from build123d import *

# Parameters (mm, degrees)
F2_R     = 3
F3_DEPTH = 50


with BuildPart() as f1:
    # F0 (on Front) → F1 (revolve)
    with BuildSketch(Plane.XZ):
        Polygon((0, 12.5), (0, 0), (22.5, 0), (22.5, 1), (10, 12.5), align=None)
        Polygon((0, 25), (0, 12.5), (10, 12.5), (16.372113, 25), align=None)
        Polygon((0, 37.5), (0, 25), (16.372113, 25), (10, 37.5), align=None)
        Polygon((0, 50), (0, 37.5), (10, 37.5), (22.5, 49), (22.5, 50), align=None)
    revolve(axis=Axis((0, 0, 25), (0, 0, 1)))

    # F2 (on face) → F3 (cut)
    with BuildSketch(Plane.XY.offset(50)):
        Circle(F2_R)
    extrude(amount=-F3_DEPTH, mode=Mode.SUBTRACT)


solid = f1.part
Design review of the part built by this model. Coordinates are the model's own, in mm. A direction names the side the tool comes from. Coordinates: 2 decimals unless noted, no trailing zeros. Loops run counter-clockwise (first coordinate to the right, second up) from the corner with the lowest first, then second, coordinate; pieces in that order, holes last. Notation, with made-up numbers: M 74,48.5 L 83,48.5 A27 cw 83,71.5 Z; hole C 61,-20.5 d5. An arc over 180 degrees is marked long. Answer as CSV lines item,"result".
Item 1: Add section D-D on z = 8.5. State the section outline as (x, y) points, plus the area to 3 significant figures.
Answer list:
outline,"C 0,0 d28.7; hole C 0,0 d6"
area,"618 mm²"
Item 2: Add section A-A on y = 0. State the section outline as (x, z) points, plus the area to 3 significant figures.
Answer list:
outline,"M -22.5,0 L -3,0 L -3,50 L -22.5,50 L -22.5,49 L -10,37.5 L -16.37,25 L -10,12.5 L -22.5,1 Z; M 3,0 L 22.5,0 L 22.5,1 L 10,12.5 L 16.37,25 L 10,37.5 L 22.5,49 L 22.5,50 L 3,50 Z"
area,"1,200 mm²"
Item 3: Add section C-C on y = 12. Count the separate pieces of the cut face and the enclosed holes in it, plus the area to 3 significant figures.
Answer list:
separate pieces,"3"
enclosed holes,"0"
area,"782 mm²"
Item 4: Machinability: for faces 1 (the face through (0, -5, 0)), 2 (the face through (-8.42, -6.45, 11.94)), which of the approach directions +Z, -Z, +X, -X, +Y, -Y give a long, thin tool a straight path to every point of the face, cutting with its end or side? Answer none if there is none.
Answer list:
face 1,"-Z, +X, -X, +Y, -Y"
face 2,"none"
Item 5: The part is to be moulded in two halves that separate along Z. For faces 3 (the face through (10.382, -19.961, 49.507)), 4 (the face through (-8.181, -6.273, 36.893)), 5 (the face through (-2.337, -10.526, 38.219)), 6 (the face through (0, -5, 50)), say which applies: pulls with the +Z half, pulls with the -Z half, needs draft (parallel to the pull), parting line crosses it, or undercut.
Answer list:
face 3,"needs draft"
face 4,"undercut"
face 5,"undercut"
face 6,"pulls with the +Z half"
Item 6: For P1, Ø1, axis at x = 5, y = -11, coming from the -Z side; P2, Ø1.5, axis at y = 1, z = 33.5, coming from the +X side; P3, Ø4, axis at y = -12, z = 34.5, coming from the -X side; P4, Ø5, axis at x = -10, z = 29.5, coming from the +Y side, all flat-tipped, find the tip position at first contact; note any pin that passes through.
Answer list:
P1,"z = 0"
P2,"x = 12.39"
P3,"x = -6.29"
P4,"y = 12.52"
Item 7: For probe 1 along Z at (x, y) = (-2, 15.5); probe 2 along Z at (x, y) = (2.5, -15.5); probe 3 along Z at (x, y) = (-10.5, -18.5), list the stretches that pass through material, from the lowest coordinate up.
Answer list:
probe 1,"0 to 7.32, 23.54 to 26.46, 42.68 to 50"
probe 2,"0 to 7.26, 23.68 to 26.32, 42.74 to 50"
probe 3,"0 to 2.13, 47.87 to 50"
